The listing builds one solid part. Answer for the finished solid, in the listing's coordinates (mm). Coordinates: 2 decimals unless noted, no trailing zeros. Write each loop counter-clockwise with the first axis right and the second up, starting at its lowest first coordinate (ties: lowest second). Pieces come first, ordered by that corner, then holes.
from build123d import *

# Parameters (mm, degrees)
BOX005_W       = 145
BOX005_H       = 110
BOX005_DEPTH   = 1
BOX006_W       = 24
BOX006_H       = 38
BOX006_DEPTH   = 1
CYLINDER_R     = 4.5
CYLINDER_DEPTH = 1
BOX002_W       = 24
BOX002_H       = 38
BOX002_DEPTH   = 1
BOX003_W       = 24
BOX003_H       = 24
BOX003_DEPTH   = 1
BOX004_W       = 24
BOX004_H       = 24
BOX004_DEPTH   = 1
BOX001_W       = 24
BOX001_H       = 38
BOX001_DEPTH   = 1
BOX_W          = 388
BOX_H          = 318
BOX_DEPTH      = 1


with BuildPart() as hueco_central:
    # Box005 → Box005 (new body)
    with BuildSketch(Plane(origin=(120, 100, 0), x_dir=(1, 0, 0), z_dir=(0, 0, 1))):
        with Locations((72.5, 55)):
            Rectangle(BOX005_W, BOX005_H)
    extrude(amount=BOX005_DEPTH)


with BuildPart() as cubo005:
    # Box006 → Box006 (new body)
    with BuildSketch(Plane(origin=(182, 280, 0), x_dir=(1, 0, 0), z_dir=(0, 0, 1))):
        with Locations((12, 19)):
            Rectangle(BOX006_W, BOX006_H)
    extrude(amount=BOX006_DEPTH)


with BuildPart() as cilindro:
    # Cylinder → Cylinder (new body)
    with BuildSketch(Plane(origin=(193.5, 235, 0), x_dir=(1, 0, 0), z_dir=(0, 0, 1))):
        Circle(CYLINDER_R)
    extrude(amount=CYLINDER_DEPTH)


with BuildPart() as cubo002:
    # Box002 → Box002 (new body)
    with BuildSketch(Plane(origin=(364, 0, 0), x_dir=(1, 0, 0), z_dir=(0, 0, 1))):
        with Locations((12, 19)):
            Rectangle(BOX002_W, BOX002_H)
    extrude(amount=BOX002_DEPTH)


with BuildPart() as cubo003:
    # Box003 → Box003 (new body)
    with BuildSketch(Plane(origin=(0, 294, 0), x_dir=(1, 0, 0), z_dir=(0, 0, 1))):
        with Locations((12, 12)):
            Rectangle(BOX003_W, BOX003_H)
    extrude(amount=BOX003_DEPTH)


with BuildPart() as cubo004:
    # Box004 → Box004 (new body)
    with BuildSketch(Plane(origin=(364, 294, 0), x_dir=(1, 0, 0), z_dir=(0, 0, 1))):
        with Locations((12, 12)):
            Rectangle(BOX004_W, BOX004_H)
    extrude(amount=BOX004_DEPTH)


with BuildPart() as obj1:
    # Box001 → Box001 (new body)
    with BuildSketch(Plane.XY):
        with Locations((12, 19)):
            Rectangle(BOX001_W, BOX001_H)
    extrude(amount=BOX001_DEPTH)

    # Fusion: union Cubo002, Cubo003, Cubo004
    add(cubo002.part)
    add(cubo003.part)
    add(cubo004.part)

    # Fusion001: union hueco central, Cubo005, Cilindro
    add(hueco_central.part)
    add(cubo005.part)
    add(cilindro.part)


with BuildPart() as cut:
    # Box → Box (new body)
    with BuildSketch(Plane.XY):
        with Locations((194, 159)):
            Rectangle(BOX_W, BOX_H)
    extrude(amount=BOX_DEPTH)

    # Cut: cut obj1
    add(obj1.part, mode=Mode.SUBTRACT)


solid = cut.part
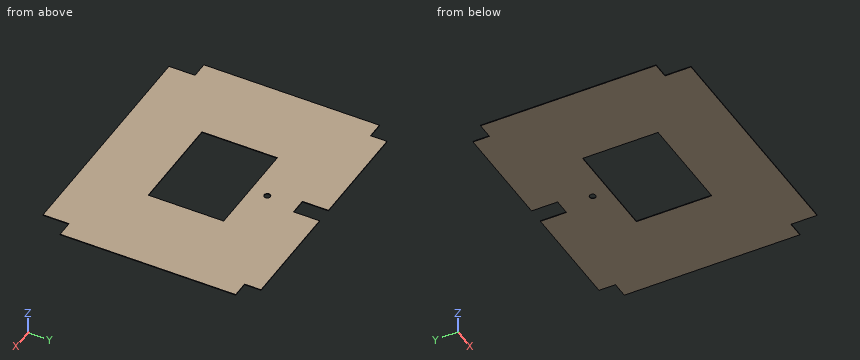
Q1. The part is cut by section A-A, the plane z = 0.5. Write down the section's boundary in (x, y), then the cut area to 3 significant figures.
Answers below:
outline: (0, 38) - (24, 38) - (24, 0) - (364, 0) - (364, 38) - (388, 38) - (388, 294) - (364, 294) - (364, 318) - (206, 318) - (206, 280) - (182, 280) - (182, 318) - (24, 318) - (24, 294) - (0, 294) - close; hole (120, 100) - (265, 100) - (265, 210) - (120, 210) - close; hole circle Ø9 at (193.5, 235)
area: 103,000 mm2
Q2. The part is cut by section C-C, the plane x = 131. Write down the section's boundary in (y, z).
Answers below:
outline: (0, 0) - (100, 0) - (100, 1) - (0, 1) - close; (210, 0) - (318, 0) - (318, 1) - (210, 1) - close
Q3. The part is cut by section D-D, the plane x = 193.5. Write down the section's boundary in (y, z), then the cut area to 3 significant figures.
Answers below:
outline: (0, 0) - (100, 0) - (100, 1) - (0, 1) - close; (210, 0) - (230.5, 0) - (230.5, 1) - (210, 1) - close; (239.5, 0) - (280, 0) - (280, 1) - (239.5, 1) - close
area: 161 mm2
Q4. Given pin 1 (0.5 mm diameter, centred on y = 25, z = 0.5, fed in from +X); pin 2 (0.5 mm diameter, centred on x = 376, z = 0.5, fed in from -Y); pin 3 (0.5 mm diameter, centred on y = 21, z = 0.5, fed in from -X), each flat-ended and moving along its own axis, determine where each tip first touches the part or whether it passes through.
Answers below:
pin 1: stops at x = 364
pin 2: stops at y = 38
pin 3: stops at x = 24
Q5. Find the intervals of material crossed by probe 1 along Y at (x, z) = (193.5, 0.45); probe 2 along Y at (x, z) = (148.5, 0.1); probe 3 along X at (y, z) = (174.5, 0.75), in increasing order.
Answers below:
probe 1: y = 0 to 100, 210 to 230.5, 239.5 to 280
probe 2: y = 0 to 100, 210 to 318
probe 3: x = 0 to 120, 265 to 388
Q6. The part is cut by section B-B, the plane y = 235. Write down the section's boundary in (x, z), then the cut area to 3 significant figures.
Answers below:
outline: (0, 0) - (189, 0) - (189, 1) - (0, 1) - close; (198, 0) - (388, 0) - (388, 1) - (198, 1) - close
area: 379 mm2
